from build123d import *

# Parameters (mm, degrees)
F0_W     = 110.5
F0_H     = 62.75
F1_DEPTH = 2
F2_W     = 12.4
F2_H     = 9.4
F3_DEPTH = 2
F4_R     = 1.625
F5_DEPTH = 2.001
F6_W     = 10
F6_H     = 43
F7_DEPTH = 5


with BuildPart() as f1:
    # F0 (on Top) → F1 (new body)
    with BuildSketch(Plane.XY):
        Rectangle(F0_W, F0_H)
    extrude(amount=F1_DEPTH)

    # F2 (on Top) → F3 (join, through all)
    with BuildSketch(Plane.XY):
        with Locations((-49.05, -36.075)):
            Rectangle(F2_W, F2_H)
    extrude(amount=F3_DEPTH)

    # F4 (on face) → F5 (cut, through all)
    with BuildSketch(Plane.XY.offset(2)):
        with Locations((-50.525, 27.25)):
            Circle(F4_R)
        with Locations((2.275, 27.25)):
            Circle(F4_R)
        with Locations((2.275, -26.7)):
            Circle(F4_R)
        with Locations((-50.525, -26.7)):
            Circle(F4_R)
    extrude(amount=-F5_DEPTH, mode=Mode.SUBTRACT)

    # F6 (on face) → F7 (join)
    with BuildSketch(Plane.XY.offset(2)):
        with Locations((50.25, 2.875)):
            Rectangle(F6_W, F6_H)
    extrude(amount=F7_DEPTH)


solid = f1.part
The listing builds one solid part. Answer for the finished solid, in the listing's coordinates (mm). A direction names the side the tool comes from. Coordinates: 2 decimals unless noted, no trailing zeros. Order: outer loops, then holes, each group sorted by start corner. A loop starts at its lowest first (then second) coordinate and runs counter-clockwise, first axis right, second up.
Q1. Consider line 1 (X direction, y = 24, z = 2.75); line 2 (Z direction, x = -37.5, y = 7); line 3 (X direction, y = 28, z = 0.5). Determine where each line is inside the solid, lowest interval first.
Q2. A cutting plane is placed at D-D, the plane z = 5. Write down the section's boundary in (x, y) (3 decimals).
Q3. Given P1, Ø5, axis at x = -50.525, y = -26.7, coming from the +Z side; P2, Ø2.5, axis at x = 50, z = 4, coming from the -Y side (3 decimals); P3, Ø1.5, axis at x = 51, z = 5.5, coming from the +Y side (3 decimals), each flat-ended and moving along its own axis, determine where each tip first touches the part or whether it passes through.
Q4. For a pull along Y with two mould halves and no side action, classify faces 5 (the face through (55.25, 0, 3)), 6 (the face through (3.776, -27.322, 1.014)), 7 (the face through (50, -18.625, 4)), 8 (the face through (-49.024, 26.628, 1.014)) as pulls with the +Y half, pulls with the -Y half, needs draft (parallel to the pull), parting line crosses it, or undercut.
Q5. A cutting plane is placed at B-B, the plane y = 5. Write down the section's boundary in (x, z).
Q6. A cutting plane is placed at C-C, the plane x = 38.5. Write down the section's boundary in (y, z) (3 decimals), and give its area (4 significant figures).
Q7. A cutting plane is placed at A-A, the plane y = -26.7. Write down the section's boundary in (x, z).
Q8. Which of the six approach directions +Z, -Z, +X, -X, +Y, -Y give full straight-line access (tool end or side, diameter ignored) to faces 1 (the face through (45.25, 3, 4)), 2 (the face through (-48.975, -26.212, 1.014)), 3 (the face through (6, -31.375, 1)), 4 (the face through (50, 24.375, 4))?
Answers follow:
1. line 1: x = 45.25 to 55.25
1. line 2: z = 0 to 2
1. line 3: x = -55.25 to -51.97, -49.08 to 0.83, 3.72 to 55.25
2. outline: (45.25, -18.625) - (55.25, -18.625) - (55.25, 24.375) - (45.25, 24.375) - close
3. P1: stops at z = 2
3. P2: stops at y = -18.625
3. P3: stops at y = 24.375
4. face 5: needs draft
4. face 6: undercut
4. face 7: pulls with the -Y half
4. face 8: undercut
5. outline: (-55.25, 0) - (55.25, 0) - (55.25, 7) - (45.25, 7) - (45.25, 2) - (-55.25, 2) - close
6. outline: (-31.375, 0) - (31.375, 0) - (31.375, 2) - (-31.375, 2) - close
6. area: 125.5 mm2
7. outline: (-55.25, 0) - (-52.15, 0) - (-52.15, 2) - (-55.25, 2) - close; (-48.9, 0) - (0.65, 0) - (0.65, 2) - (-48.9, 2) - close; (3.9, 0) - (55.25, 0) - (55.25, 2) - (3.9, 2) - close
8. face 1: +Z, -X, +Y, -Y
8. face 2: +Z, -Z
8. face 3: +Z, -Z, +X, -Y
8. face 4: +Z, +X, -X, +Y
